```python
from build123d import *

# Parameters (mm, degrees)
SKETCH_1_W          = 457.2
SKETCH_1_H          = 76.2
EXTRUDE_1_DEPTH     = 101.6
SKETCH_1_3_W        = 73.2
SKETCH_1_3_H        = 72.2
SKETCH_1_3_W_2      = 74.2
CUT_EXTRUDE_1_DEPTH = 102.6


with BuildPart() as part:
    # Эскиз1 → Бобышка-Вытянуть1 (new body)
    with BuildSketch(Plane.XY):
        Rectangle(SKETCH_1_W, SKETCH_1_H)
    extrude(amount=EXTRUDE_1_DEPTH)

    # Эскиз1<3> → Вырез-Вытянуть1 (cut, through all)
    with BuildSketch(Plane.XY):
        with Locations((-190, 0)):
            Rectangle(SKETCH_1_3_W, SKETCH_1_3_H)
        with Locations((-114.3, 0)):
            Rectangle(SKETCH_1_3_W_2, SKETCH_1_3_H)
        with Locations((-38.1, 0)):
            Rectangle(SKETCH_1_3_W_2, SKETCH_1_3_H)
        with Locations((38.1, 0)):
            Rectangle(SKETCH_1_3_W_2, SKETCH_1_3_H)
        with Locations((114.3, 0)):
            Rectangle(SKETCH_1_3_W_2, SKETCH_1_3_H)
        with Locations((190, 0)):
            Rectangle(SKETCH_1_3_W, SKETCH_1_3_H)
    extrude(amount=CUT_EXTRUDE_1_DEPTH, mode=Mode.SUBTRACT)


solid = part.part
```
Check sheet for the modelled part. Datum: model origin and axes. Units: mm. A direction names the side the tool comes from. Give positions to 0.01 mm unless a question says otherwise; leave off trailing zeros. Write each loop counter-clockwise with the first axis right and the second up, starting at its lowest first coordinate (ties: lowest second). Pieces come first, ordered by that corner, then holes. Notation, with made-up numbers: (81, -25) -> (107, -25) arc R29 ccw to (107, 11) -> close; hole circle Ø10 at (70, 35). An arc over 180 degrees is marked (long way). Use CSV: the item, a comma, the result in double quotes. Start each with the question number.
Q1. Cross-section at B-B on z = 43. Enter the section's corners in (x, y).
Q2. Cross-section at A-A on y = 25. Enter the section's corners in (x, z).
Q3. Cross-section at C-C on x = -66. Enter the section's corners in (y, z).
Q4. Tool access check on faces 4 (the flat face through (-1, 37, 0)), 5 (the flat face through (-115, 36.1, 50)). Record the directions out of +Z, -Z, +X, -X, +Y, -Y that give a thin tool (end or side, any length) a straight path to the whole face; none if there is none.
Q5. Scan line: line 1 along Y through (x, z) = (106, 79.5). Record every from-to range of solid material in increasing order.
Q6. Release check for a two-part mould opening along Y. For faces 1 (the flat face through (-228.6, -1, 50)), 2 (the flat face through (-77.2, -1, 50)), 3 (the flat face through (-3, -38.1, 50)) record: +Y half, -Y half, draft (parallel to the pull), parting line (faces both ways), or undercut.
Working result:
1,outline,"(-228.6, -38.1) -> (228.6, -38.1) -> (228.6, 38.1) -> (-228.6, 38.1) -> close; hole (-226.6, -36.1) -> (-153.4, -36.1) -> (-153.4, 36.1) -> (-226.6, 36.1) -> close; hole (-151.4, -36.1) -> (-77.2, -36.1) -> (-77.2, 36.1) -> (-151.4, 36.1) -> close; hole (-75.2, -36.1) -> (-1, -36.1) -> (-1, 36.1) -> (-75.2, 36.1) -> close; hole (1, -36.1) -> (75.2, -36.1) -> (75.2, 36.1) -> (1, 36.1) -> close; hole (77.2, -36.1) -> (151.4, -36.1) -> (151.4, 36.1) -> (77.2, 36.1) -> close; hole (153.4, -36.1) -> (226.6, -36.1) -> (226.6, 36.1) -> (153.4, 36.1) -> close"
2,outline,"(-228.6, 0) -> (-226.6, 0) -> (-226.6, 101.6) -> (-228.6, 101.6) -> close; (-153.4, 0) -> (-151.4, 0) -> (-151.4, 101.6) -> (-153.4, 101.6) -> close; (-77.2, 0) -> (-75.2, 0) -> (-75.2, 101.6) -> (-77.2, 101.6) -> close; (-1, 0) -> (1, 0) -> (1, 101.6) -> (-1, 101.6) -> close; (75.2, 0) -> (77.2, 0) -> (77.2, 101.6) -> (75.2, 101.6) -> close; (151.4, 0) -> (153.4, 0) -> (153.4, 101.6) -> (151.4, 101.6) -> close; (226.6, 0) -> (228.6, 0) -> (228.6, 101.6) -> (226.6, 101.6) -> close"
3,outline,"(-38.1, 0) -> (-36.1, 0) -> (-36.1, 101.6) -> (-38.1, 101.6) -> close; (36.1, 0) -> (38.1, 0) -> (38.1, 101.6) -> (36.1, 101.6) -> close"
4,face 4,"-Z, +X, -X, +Y, -Y"
4,face 5,"+Z, -Z"
5,line 1,"y = -38.1 to -36.1, 36.1 to 38.1"
6,face 1,"draft"
6,face 2,"undercut"
6,face 3,"-Y half"
